Autodesk Inventor part; units mm, degrees
ref_plane "YZ Plane" through (0, 0, 0) normal (1, 0, 0) x (0, 1, 0)
ref_plane "XZ Plane" through (0, 0, 0) normal (0, 1, 0) x (-1, 0, 0)
ref_plane "XY Plane" through (0, 0, 0) normal (0, 0, 1) x (1, 0, 0)
sketch "Sketch1" plane through (0, 0, 0) normal (1, 0, 0) x (0, 1, 0)
  line L0 (0, 0) -> (0, -112)
  line L1 (0, -112) -> (3, -112)
  line L2 (3, -112) -> (3, 0)
  line L3 (3, 0) -> (0, 0)
  line L4 (3, 0) -> (3, -6)
  line L5 (3, -112) -> (3, -106)
  line L6 (3, -112) -> (5, -112)
  line L7 (5, -112) -> (5, -106)
  line L8 (5, -106) -> (3, -106)
  line L9 (3, 0) -> (5, 0)
  line L10 (5, 0) -> (5, -6)
  line L11 (5, -6) -> (3, -6)
  line L12 (3, -106) -> (0.5, -106)
  line L13 (0.5, -106) -> (0.5, -6)
  line L14 (0.5, -6) -> (3, -6)
  line L15 (5, -6) -> (5, -7)
  line L16 (5, -7) -> (0.5, -7)
  line L17 (5, -106) -> (5, -105)
  line L18 (5, -105) -> (0.5, -105)
  line L19 (3, -7) -> (3.1, -7)
  line L20 (2.5, -7) -> (2.5, -105)
  point P0 (3, -105)
  point P1 (2, -6)
  point P2 (3.1, -105)
  dimension "d0" = 112
  dimension "d1" = 3
  dimension "d2" = 6
  dimension "d3" = 6
  dimension "d5" = 2
  dimension "d6" = 2
  dimension "d7" = 2.5
  dimension "d8" = 1
  dimension "d9" = 1
  dimension "d22" = 2
revolve "Revolution1" add sketch "Sketch1" angle 360 about axis through (0, 0, 0) along (0, 0, -1) contours L9 L10 L11 L2 | L2 L8 L7 L6 | L11 L15 L16 L2 | L2 L16 L13 L14 | L12 L13 L18 L2 | L2 L18 L17 L8 | L20 L18 L13 L16
thread "Thread1"
thread "Thread2"
chamfer "Chamfer1" distance 0.5 angle 45 2 edges at (0, -3, 0) (0, -3, -112)
chamfer "Chamfer2" distance 0.5 angle 45 4 edges at (0, -5, -112) (0, -5, -105) (0, -5, -7) (0, -5, 0)
chamfer "Chamfer3" distance 2 angle 45 2 edges at (0, -2.5, -7) (0, -2.5, -105)
properties part number "Heater"
Design review of the part built by this model. Coordinates are the model's own, in mm. A direction names the side the tool comes from. Give positions to 0.01 mm unless a question says otherwise; leave off trailing zeros. Write each loop counter-clockwise with the first axis right and the second up, starting at its lowest first coordinate (ties: lowest second). Pieces come first, ordered by that corner, then holes. Notation, with made-up numbers: (39, 32.5) - (96, 32.5) arc R25 cw to (96, 63.5) - close; hole circle Ø7 at (60, -4.5). An arc over 180 degrees is marked (long way). Return JSON: item names as keys, results as strings. Group by question number.
(1) Mouldability with a two-part tool opening along Y and no side actions: class faces 1 (the flat face through (0, 1, -6)), 2 (the cylindrical face through (0, -3, -109)), 3 (the conical face through (-2.563, -0.569, -103.126)), 4 (the flat face through (-4, 0, -112)) as +Y half, -Y half, draft (parallel to the pull), parting line (faces both ways), or undercut.
(2) We need section A-A, the plane z = -67. Give the boundary of the cut face in (x, y).
(3) To check wall thickness, follow probe 1 along X at (y, z) = (0, -2.2); probe 2 along Z at (x, y) = (1.5, 1.25); probe 3 along X at (y, z) = (-1.75, -107). State the ranges of each line that lie inside material, in increasing order.
(4) Machinability: for faces 5 (the conical face through (2.563, -0.569, -8.874)), 6 (the flat face through (0, 1, -106)), 7 (the cylindrical face through (0, -3, -3)), which of the approach directions +Z, -Z, +X, -X, +Y, -Y give a long, thin tool a straight path to every point of the face, cutting with its end or side? Answer none if there is none.
(5) Insertion check: pin 1 (5 mm diameter, centred on y = 4, z = -54, fed in from -X); pin 2 (4 mm diameter, centred on x = -1, y = 0.5, fed in from -Z); pin 3 (3.5 mm diameter, centred on x = 0, y = 0, fed in from -Z). Each pin has a flat end and moves straight along its axis. Give the tip position at first contact, or say it passes through.
Reported:
{
 "1": {"face 1": "undercut", "face 2": "undercut", "face 3": "parting line", "face 4": "draft"},
 "2": {"outline": "circle Ø5 at (0, 0); hole circle Ø1 at (0, 0)"},
 "3": {"probe 1": "x = -5 to -3, 3 to 5", "probe 2": "z = -106 to -6", "probe 3": "x = -4.68 to -2.44, 2.44 to 4.68"},
 "4": {"face 5": "none", "face 6": "-Z", "face 7": "+Z"},
 "5": {"pin 1": "stops at x = -2", "pin 2": "stops at z = -111.62", "pin 3": "stops at z = -106"}
}
